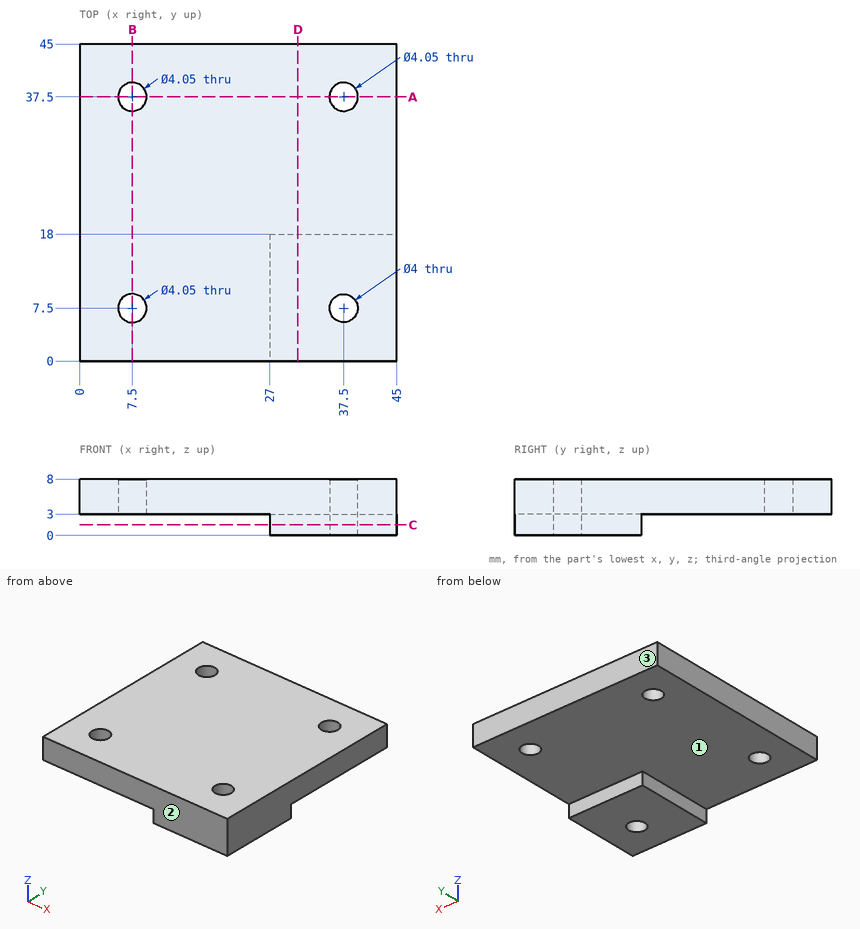
Print and shaded views of the part. All mm, measured from the part's lowest x, y and z. Round coordinates to 2 decimals unless told otherwise and drop trailing zeros. Order: outer loops, then holes, each group sorted by start corner. A loop starts at its lowest first (then second) coordinate and runs counter-clockwise, first axis right, second up. Notation, with made-up numbers: (39, 11) - (75, 11) arc R22 ccw to (75, 25) - close; hole circle Ø3 at (-37, 51.5). An arc over 180 degrees is marked (long way). Use a Markdown table: item, result.
1) Flat gauge pins, fed straight in: pin 1 Ø1.5 at (y, z) = (27.5, 3) entering from -X; pin 2 Ø4.5 at (x, y) = (7.5, 37.5) entering from -Z; pin 3 Ø1.5 at (x, z) = (39.5, 1) entering from +Y; pin 4 Ø2.5 at (x, y) = (37.5, 37.5) entering from -Z. Where does each tip first touch, or does it go through?
Recorded:
| item | result |
|---|---|
| pin 1 | stops at x = 0 |
| pin 2 | stops at z = 3 |
| pin 3 | stops at y = 18 |
| pin 4 | passes through |
2) Saw through at D-D on x = 31. Write the cut outline in (y, z), and give its area (3 significant figures).
Recorded:
| item | result |
|---|---|
| outline | (0, 0) - (18, 0) - (18, 3) - (45, 3) - (45, 8) - (0, 8) - close |
| area | 279 mm² |
3) Saw through at C-C on z = 1.5. Write the cut outline in (x, y).
Recorded:
| item | result |
|---|---|
| outline | (27, 0) - (45, 0) - (45, 18) - (27, 18) - close; hole circle Ø4 at (37.5, 7.5) |
4) Pull direction Y, two halves, no side cores. Call the marked faces 1, 2 and 3: pulls with the +Y half, pulls with the -Y half, needs draft (parallel to the pull), parting line crosses it, or undercut.
Recorded:
| item | result |
|---|---|
| face 1 | needs draft |
| face 2 | pulls with the -Y half |
| face 3 | pulls with the +Y half |
5) Saw through at A-A on y = 37.5. Write the cut outline in (x, z) (3 decimals).
Recorded:
| item | result |
|---|---|
| outline | (0, 3) - (5.475, 3) - (5.475, 8) - (0, 8) - close; (9.525, 3) - (35.475, 3) - (35.475, 8) - (9.525, 8) - close; (39.525, 3) - (45, 3) - (45, 8) - (39.525, 8) - close |
6) Wall check: L1, parallel to Y at x = 37.5, z = 4 (3 decimals); L2, parallel to Y at x = 33, z = 1.5; L3, parallel to Y at x = 37, z = 4.5. Give the ranges that are in metal, low to high.
Recorded:
| item | result |
|---|---|
| L1 | y = 0 to 5.5, 9.5 to 35.475, 39.525 to 45 |
| L2 | y = 0 to 18 |
| L3 | y = 0 to 5.56, 9.44 to 35.54, 39.46 to 45 |
